The model under review builds one solid part; all positions refer to its coordinate system, in mm. Face numbers are marked on the shaded views. A direction names the side the tool comes from. Coordinates: 2 decimals unless noted, no trailing zeros. Write each loop counter-clockwise with the first axis right and the second up, starting at its lowest first coordinate (ties: lowest second). Pieces come first, ordered by that corner, then holes.
1) For line 1 (X direction, y = 0, z = 1); line 2 (X direction, y = 0, z = 1.55), list the stretches that pass through material, from the lowest coordinate up.
2) Machinability: for the marked faces 1 and 2, which of the approach directions +Z, -Z, +X, -X, +Y, -Y give a long, thin tool a straight path to every point of the face, cutting with its end or side? Answer none if there is none.
3) Add section A-A, the plane x = 0. State the section outline as (y, z) points (3 decimals), then the cut area to 3 significant figures.
4) Add section C-C, the plane z = 1.75. State the section outline as (x, y) points, then the cut area to 3 significant figures.
5) Add section B-B, the plane y = -12. State the section outline as (x, z) points.
6) Add section D-D, the plane y = -2.75. State the section outline as (x, z) points, then the cut area to 3 significant figures.
7) For P1, Ø1.1, axis at x = 0.5, z = 3, coming from the -Y side (3 decimals); P2, Ø13, axis at x = 6.5, y = 6, coming from the -Z side; P3, Ø0.5, axis at x = 1.5, y = -14, coming from the +Z side; P4, Ø1, axis at x = 4, z = 1.5, coming from the +Y side, all flat-tipped, find the tip position at first contact; note any pin that passes through.
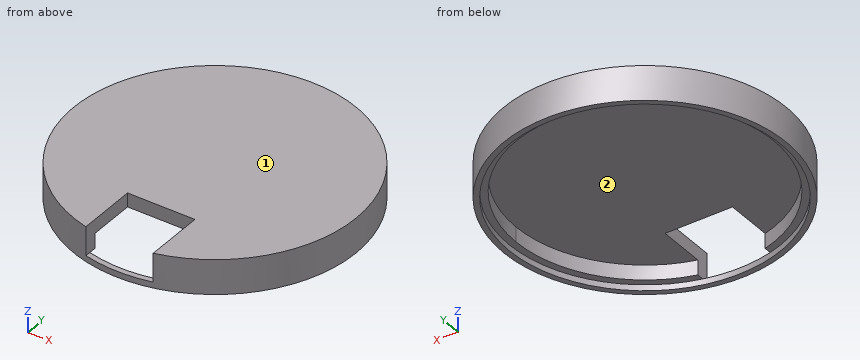
from build123d import *

# Parameters (mm, degrees)
F0_R     = 13.5
F0_W     = 6
F0_H     = 4.25
F1_DEPTH = 1.2
F2_DEPTH = 4.2
F3_R     = 14.25
F3_R_2   = 13.7
F3_R_3   = 13.5
F4_DEPTH = 2.9
F5_DEPTH = 0.6
F3_W     = 6
F3_H     = 4.25
F6_DEPTH = 1.5
F7_W     = 6.8
F7_H     = 3
F8_DEPTH = 8


with BuildPart() as f1:
    # F0 (on Top) → F1 (new body)
    with BuildSketch(Plane.XY):
        Circle(F0_R)
        with Locations((0, -10.295)):
            Rectangle(F0_W, F0_H, mode=Mode.SUBTRACT)
        with Locations((0, -10.295)):
            Rectangle(F0_W, F0_H)
    extrude(amount=F1_DEPTH)

    # F0 (on Top) → F2 (join)
    with BuildSketch(Plane.XY):
        with Locations((0, -10.295)):
            Rectangle(F0_W, F0_H)
    extrude(amount=F2_DEPTH)


with BuildPart() as f4:
    # F3 (on face) → F4 (new body)
    with BuildSketch(Plane.XY.offset(1.2)):
        Circle(F3_R)
        Circle(F3_R_2, mode=Mode.SUBTRACT)
        Circle(F3_R_2)
        Circle(F3_R_3, mode=Mode.SUBTRACT)
        Circle(F3_R_3)
        with BuildLine():
            Line((3.4, -12.5475097131), (3.4, -12.795))
            Line((3.4, -12.795), (2.2995597405, -12.795))
            ThreePointArc((2.2995597405, -12.795), (0, -13), (-2.2995597405, -12.795))
            Line((-2.2995597405, -12.795), (-3.4, -12.795))
            Line((-3.4, -12.795), (-3.4, -12.5475097131))
            ThreePointArc((-3.4, -12.5475097131), (-7.8993670633, 10.3247275993), (13, 0))
            ThreePointArc((13, 0), (10.3247275993, -7.8993670633), (3.4, -12.5475097131))
        make_face(mode=Mode.SUBTRACT)
        with BuildLine():
            Line((3.4, -7.795), (3.4, -12.5475097131))
            ThreePointArc((3.4, -12.5475097131), (10.3247275993, -7.8993670633), (13, 0))
            ThreePointArc((13, 0), (-7.8993670633, 10.3247275993), (-3.4, -12.5475097131))
            Line((-3.4, -12.5475097131), (-3.4, -7.795))
            Line((-3.4, -7.795), (3.4, -7.795))
        make_face()
        with BuildLine():
            ThreePointArc((-2.2995597405, -12.795), (0, -13), (2.2995597405, -12.795))
            Line((2.2995597405, -12.795), (-2.2995597405, -12.795))
        make_face()
    extrude(amount=F4_DEPTH)

    # F3 (on face) → F5 (join)
    with BuildSketch(Plane.XY.offset(1.2)):
        Circle(F3_R)
        Circle(F3_R_2, mode=Mode.SUBTRACT)
    extrude(amount=-F5_DEPTH)

    # F3 (on face) → F6 (cut)
    with BuildSketch(Plane.XY.offset(1.2)):
        with BuildLine():
            Line((3.4, -7.795), (3.4, -12.5475097131))
            ThreePointArc((3.4, -12.5475097131), (10.3247275993, -7.8993670633), (13, 0))
            ThreePointArc((13, 0), (-7.8993670633, 10.3247275993), (-3.4, -12.5475097131))
            Line((-3.4, -12.5475097131), (-3.4, -7.795))
            Line((-3.4, -7.795), (3.4, -7.795))
        make_face()
        with BuildLine():
            Line((-2.2995597405, -12.795), (2.2995597405, -12.795))
            ThreePointArc((2.2995597405, -12.795), (2.8524652793, -12.6831952532), (3.4, -12.5475097131))
            Line((3.4, -12.5475097131), (3.4, -7.795))
            Line((3.4, -7.795), (-3.4, -7.795))
            Line((-3.4, -7.795), (-3.4, -12.5475097131))
            ThreePointArc((-3.4, -12.5475097131), (-2.8524652793, -12.6831952532), (-2.2995597405, -12.795))
        make_face()
        with Locations((0, -10.295)):
            Rectangle(F3_W, F3_H, mode=Mode.SUBTRACT)
        with BuildLine():
            ThreePointArc((-2.2995597405, -12.795), (0, -13), (2.2995597405, -12.795))
            Line((2.2995597405, -12.795), (-2.2995597405, -12.795))
        make_face()
    extrude(amount=F6_DEPTH, mode=Mode.SUBTRACT)

    # F7 (on face) → F8 (cut)
    with BuildSketch(Plane.XZ.offset(12.42)):
        with Locations((0, 2.7)):
            Rectangle(F7_W, F7_H)
    extrude(amount=F8_DEPTH, mode=Mode.SUBTRACT)


solid = f4.part
Geometry results:
1. line 1: x = -14.25 to -13.7, 13.7 to 14.25
1. line 2: x = -14.25 to -13, 13 to 14.25
2. face 1: +Z, +X, -X, +Y, -Y
2. face 2: -Z
3. outline: (-14.25, 0.6) - (-13.7, 0.6) - (-13.7, 1.2) - (-14.25, 1.2) - close; (-7.795, 2.7) - (13, 2.7) - (13, 1.2) - (13.7, 1.2) - (13.7, 0.6) - (14.25, 0.6) - (14.25, 4.1) - (-7.795, 4.1) - close
3. area: 33.4 mm2
4. outline: (-3.4, -13.84) - (-3.4, -12.55) arc R13 cw (long way) to (3.4, -12.55) - (3.4, -13.84) arc R14.25 ccw (long way) to start
4. area: 98.4 mm2
5. outline: (-7.69, 0.6) - (-6.61, 0.6) - (-6.61, 1.2) - (-5, 1.2) - (-5, 2.7) - (-3.4, 2.7) - (-3.4, 4.1) - (-7.69, 4.1) - close; (3.4, 2.7) - (5, 2.7) - (5, 1.2) - (6.61, 1.2) - (6.61, 0.6) - (7.69, 0.6) - (7.69, 4.1) - (3.4, 4.1) - close
6. outline: (-13.98, 0.6) - (-13.42, 0.6) - (-13.42, 1.2) - (-12.71, 1.2) - (-12.71, 2.7) - (12.71, 2.7) - (12.71, 1.2) - (13.42, 1.2) - (13.42, 0.6) - (13.98, 0.6) - (13.98, 4.1) - (-13.98, 4.1) - close
6. area: 43.7 mm2
7. P1: stops at y = -7.795
7. P2: stops at z = 0.6
7. P3: stops at z = 1.2
7. P4: stops at y = 13.81
